Part model, mm, in its own coordinate system. Face numbers are marked on the shaded views. A direction names the side the tool comes from. Round coordinates to 2 decimals unless told otherwise and drop trailing zeros. Loops run counter-clockwise (first coordinate to the right, second up) from the corner with the lowest first, then second, coordinate; pieces in that order, holes last. Notation, with made-up numbers: M 63,22 L 108,22 A17 ccw 108,36 Z; hole C 28,-27.75 d7. An arc over 180 degrees is marked long. Answer as CSV lines item,"result". Start each with the question number.
Item 1: Wall check: line 1 (Z direction, x = -48.5, y = -39); line 2 (Z direction, x = 6, y = -33.5); line 3 (X direction, y = -113.5, z = 15). Give the ranges that are in metal, low to high.
Item 2: Which spindle directions (+Z, -Z, +X, -X, +Y, -Y) get a long thin tool onto all of the face, cutting with end or side? Do the marked faces 5, 6 and 7. Say none if no direction does.
Item 3: Band-saw the part on B-B (x = 0). Give the cut face in (y, z).
Item 4: Band-saw the part on C-C (z = 52.5). Give the cut face in (x, y), and give its area (3 significant figures).
Item 5: Mould opens along Z. For the marked faces 1, 2, 3 and 4 say: pulls with the +Z half, pulls with the -Z half, needs draft (parallel to the pull), parting line crosses it, or undercut.
Item 6: Band-saw the part on A-A (z = -26.5). Give the cut face in (x, y).
Item 7: Drop flat-ended pins along their axis: pin 1 Ø8 at (y, z) = (-33, 51.5) entering from +X; pin 2 Ø8.5 at (x, y) = (58.64, -116.69) entering from +Z; pin 3 Ø5 at (x, y) = (-59.53, -116.69) entering from -Z. Give the stop position or say it passes through.
Item 8: Band-saw the part on D-D (y = -99). Count the separate pieces of the cut face and the enclosed holes in it, and give its area (3 significant figures).
```python
from build123d import *

# Parameters (mm, degrees)
F0_W     = 127
F0_H     = 32.3606841266
F0_H_2   = 26.7147784284
F1_DEPTH = 127
F2_R     = 5.08
F3_R     = 2.1310745611
F4_DEPTH = 25.4
F5_R     = 2.6680723022
F6_DEPTH = 25.4
F7_R     = 42.1805785401
F7_R_2   = 34.8133831429
F8_DEPTH = 25.4
F9_DEPTH = 25.4
F10_R    = 5.08


with BuildPart() as f1:
    # F0 (on Front) → F1 (new body)
    with BuildSketch(Plane.XZ):
        with BuildLine():
            ThreePointArc((69.8099806905, 32.3913091956), (67.950108751, 36.8814372561), (63.4599806905, 38.7413091956))
            Line((63.4599806905, 38.7413091956), (-63.4599806905, 38.7413091956))
            ThreePointArc((-63.4599806905, 38.7413091956), (-67.950108751, 36.8814372561), (-69.8099806905, 32.3913091956))
            Line((-69.8099806905, 32.3913091956), (-69.8099806905, -38.7413091956))
            Line((-69.8099806905, -38.7413091956), (69.8099806905, -38.7413091956))
            Line((69.8099806905, -38.7413091956), (69.8099806905, 32.3913091956))
        make_face()
        with Locations((-0.0400193095, -16.1803420633)):
            Rectangle(F0_W, F0_H, mode=Mode.SUBTRACT)
        with Locations((-0.0400193095, 19.0339199814)):
            Rectangle(F0_W, F0_H_2, mode=Mode.SUBTRACT)
    extrude(amount=F1_DEPTH)

    # F2
    f2_edges = [f1.edges().sort_by_distance(p)[0] for p in [
        (69.809981, -127, -3.175),
        (67.950109, -127, 36.881437),
        (0, -127, 38.741309),
        (-67.950109, -127, 36.881437),
        (-69.809981, -127, -3.175),
        (69.809981, 0, -3.175),
        (67.950109, 0, 36.881437),
        (0, 0, 38.741309),
        (-67.950109, 0, 36.881437),
        (-69.809981, 0, -3.175),
    ]]
    fillet(f2_edges, radius=F2_R)

    # F3 (on face) → F4 (cut)
    with BuildSketch(Plane(origin=(0, 0, -38.7413091956), x_dir=(1, 0, 0), z_dir=(0, 0, -1))):
        with Locations((-42.0244000852, 79.0478363633)):
            Circle(F3_R)
        with Locations((-42.0244000852, 50.4565563633)):
            Circle(F3_R)
        with Locations((39.2230374546, 79.047831549)):
            Circle(F3_R)
        with Locations((39.2230374546, 50.456551549)):
            Circle(F3_R)
    extrude(amount=-F4_DEPTH, mode=Mode.SUBTRACT)

    # F5 (on face) → F6 (cut)
    with BuildSketch(Plane(origin=(0, 0, -38.7413091956), x_dir=(1, 0, 0), z_dir=(0, 0, -1))):
        with Locations((-59.5310516655, 116.688169539)):
            Circle(F5_R)
        with Locations((-59.98695, 10.82233)):
            Circle(F5_R)
        with Locations((58.6440783345, 116.688169539)):
            Circle(F5_R)
        with Locations((58.18818, 10.82233)):
            Circle(F5_R)
    extrude(amount=-F6_DEPTH, mode=Mode.SUBTRACT)

    # F7 (on face) → F8 (join)
    with BuildSketch(Plane.XY.offset(38.7413091956)):
        with Locations((0, -61.0473752022)):
            Circle(F7_R)
        with Locations((0, -61.0473752022)):
            Circle(F7_R_2, mode=Mode.SUBTRACT)
    extrude(amount=F8_DEPTH)

    # F9 (cut): a face of the model
    f9_faces = [f1.faces().sort_by_distance(p)[0] for p in [
        (0, -61.0473752022, 38.7413091956),
    ]]
    extrude(f9_faces, amount=-F9_DEPTH, mode=Mode.SUBTRACT)

    # F10
    f10_edges = [f1.edges().sort_by_distance(p)[0] for p in [
        (-34.813383, -61.047375, 32.391309),
    ]]
    fillet(f10_edges, radius=F10_R)


solid = f1.part
```
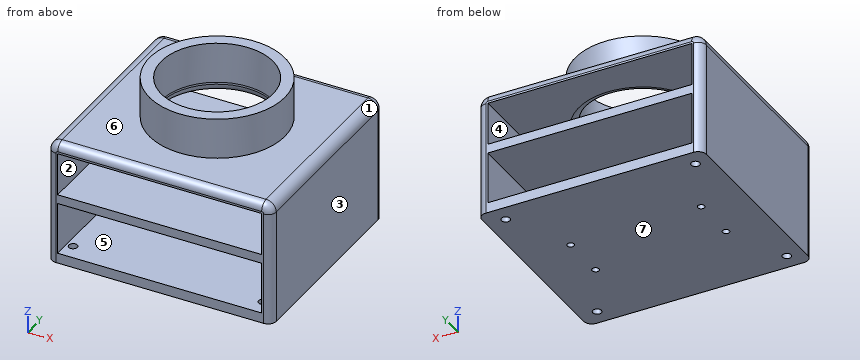
Answer block:
1,line 1,"z = -38.74 to -32.36, 0 to 5.68, 32.39 to 38.74"
1,line 2,"z = -38.74 to -32.36, 0 to 5.68"
1,line 3,"x = -69.81 to -63.54, 63.46 to 69.81"
2,face 5,"+Y, -Y"
2,face 6,"+Z"
2,face 7,"-Z, +X, -X, +Y, -Y"
3,outline,"M -127,-38.74 L 0,-38.74 L 0,-32.36 L -127,-32.36 Z; M -127,0 L 0,0 L 0,5.68 L -127,5.68 Z; M -127,32.39 L -100.94,32.39 A5.08 ccw -95.86,37.47 L -95.86,64.14 L -103.23,64.14 L -103.23,38.74 L -121.92,38.74 A5.08 ccw -127,33.66 Z; M -26.23,37.47 A5.08 ccw -21.15,32.39 L 0,32.39 L 0,33.66 A5.08 ccw -5.08,38.74 L -18.87,38.74 L -18.87,64.14 L -26.23,64.14 Z"
4,outline,"C 0,-61.05 d84.36; hole C 0,-61.05 d69.63"
4,area,"1,780 mm^2"
5,face 1,"pulls with the +Z half"
5,face 2,"undercut"
5,face 3,"needs draft"
5,face 4,"undercut"
6,outline,"M -69.81,-121.92 A5.08 ccw -64.73,-127 L -63.54,-127 L -63.54,0 L -64.73,0 A5.08 ccw -69.81,-5.08 Z; M 63.46,-127 L 64.73,-127 A5.08 ccw 69.81,-121.92 L 69.81,-5.08 A5.08 ccw 64.73,0 L 63.46,0 Z"
7,pin 1,"stops at x = 34.65"
7,pin 2,"stops at z = 38.74"
7,pin 3,"stops at z = 0"
8,separate pieces,"1"
8,enclosed holes,"2"
8,area,"4,230 mm^2"
